Can you work these out from the model? Positions are in its coordinate system, mm. Give positions to 0.01 mm unless a question says otherwise; leave off trailing zeros. Loops run counter-clockwise (first coordinate to the right, second up) from the corner with the lowest first, then second, coordinate; pieces in that order, holes last. Notation, with made-up numbers: (33.25, -40) -> (66.25, -40) arc R23 ccw to (66.25, -16) -> close; hole circle Ø9 at (-33, 39.5). An arc over 180 degrees is marked (long way). One line per question, with ' | ' between items.
from build123d import *

# Parameters (mm, degrees)
F0_R      = 0.635
F1_DEPTH  = 3.175
F2_W      = 508
F2_H      = 25.4
F3_DEPTH  = 6.35
F4_W      = 25.4
F4_H      = 63.5
F4_H_2    = 152.4
F5_DEPTH  = 6.35
F6_W      = 508
F6_H      = 25.4
F7_DEPTH  = 6.35
F8_W      = 152.4
F8_H      = 25.4
F9_DEPTH  = 6.35
F10_W     = 25.4
F10_H     = 152.4
F11_DEPTH = 6.35
F12_W     = 25.4
F12_H     = 152.4
F13_DEPTH = 6.35
F14_W     = 76.2
F14_H     = 25.4
F15_DEPTH = 6.35


# Not quite as in the source:
# - a feature of the source that left no trace in its solid (it failed there, or was rolled back) is left out


with BuildPart() as f1:
    # F0 (on Top) → F1 (new body)
    with BuildSketch(Plane.XY):
        Polygon((285.75, -298.45), (323.85, -298.45), (577.85, -298.45), (615.95, -298.45), (1187.45, -298.45), (1276.35, -298.45), (1276.35, 298.45), (1187.45, 298.45), (285.75, 298.45), (285.75, 349.25), (361.95, 349.25), (361.95, 577.85), (285.75, 577.85), (285.75, 704.85), (-285.75, 704.85), (-285.75, 577.85), (-361.95, 577.85), (-361.95, 349.25), (-285.75, 349.25), (-285.75, 336.55), (-285.75, 298.45), (-323.85, 298.45), (-361.95, 298.45), (-577.85, 298.45), (-577.85, -298.45), (-323.85, -298.45), (-285.75, -298.45), (-285.75, -336.55), (-285.75, -622.3), (-25.4, -622.3), (-25.4, -774.7), (25.4, -774.7), (25.4, -622.3), (177.8, -622.3), (285.75, -622.3), (285.75, -336.55), align=None)
        with Locations((0, -463.55)):
            Circle(F0_R, mode=Mode.SUBTRACT)
        with Locations((-450.85, 0)):
            Circle(F0_R, mode=Mode.SUBTRACT)
        Circle(F0_R, mode=Mode.SUBTRACT)
        with Locations((0, 463.55)):
            Circle(F0_R, mode=Mode.SUBTRACT)
        with Locations((450.85, 0)):
            Circle(F0_R, mode=Mode.SUBTRACT)
        with Locations((812.8, 0)):
            Circle(F0_R, mode=Mode.SUBTRACT)
        with Locations((901.7, 0)):
            Circle(F0_R, mode=Mode.SUBTRACT)
        with Locations((990.6, 0)):
            Circle(F0_R, mode=Mode.SUBTRACT)
    extrude(amount=F1_DEPTH)

    # F2 (on face) → F3 (join)
    with BuildSketch(Plane.XY.offset(3.175)):
        with Locations((0, 679.45)):
            Rectangle(F2_W, F2_H)
    extrude(amount=F3_DEPTH)

    # F4 (on face) → F5 (join)
    with BuildSketch(Plane.XY.offset(3.175)):
        with Locations((0, -679.45)):
            Rectangle(F4_W, F4_H)
        with Locations((-323.85, 463.55)):
            Rectangle(F4_W, F4_H_2)
        with Locations((323.85, 463.55)):
            Rectangle(F4_W, F4_H_2)
    extrude(amount=F5_DEPTH)

    # F6 (on face) → F7 (join)
    with BuildSketch(Plane(origin=(0, 0, 0), x_dir=(1, 0, 0), z_dir=(0, 0, -1))):
        with Locations((901.7, -247.65)):
            Rectangle(F6_W, F6_H)
    extrude(amount=F7_DEPTH)

    # F8 (on face) → F9 (join)
    with BuildSketch(Plane(origin=(0, 0, 0), x_dir=(1, 0, 0), z_dir=(0, 0, -1))):
        with Locations((450.85, -260.35)):
            Rectangle(F8_W, F8_H)
        with Locations((-450.85, -260.35)):
            Rectangle(F8_W, F8_H)
    extrude(amount=F9_DEPTH)

    # F10 (on face) → F11 (join)
    with BuildSketch(Plane.XY.offset(3.175)):
        with Locations((1250.95, 152.4)):
            Rectangle(F10_W, F10_H)
        with Locations((1250.95, -152.4)):
            Rectangle(F10_W, F10_H)
    extrude(amount=F11_DEPTH)

    # F12 (on face) → F13 (join)
    with BuildSketch(Plane.XY):
        with Locations((-552.45, 152.4)):
            Rectangle(F12_W, F12_H)
        with Locations((-552.45, -152.4)):
            Rectangle(F12_W, F12_H)
    extrude(amount=-F13_DEPTH)

    # F14 (on face) → F15 (join)
    with BuildSketch(Plane(origin=(0, 0, 0), x_dir=(1, 0, 0), z_dir=(0, 0, -1))):
        with Locations((901.7, 247.65)):
            Rectangle(F14_W, F14_H)
    extrude(amount=F15_DEPTH)


solid = f1.part
Q1. If I drill on probe 1 along Y at (x, z) = (812.8, 1.2) (3 decimals); probe 2 along Y at (x, z) = (0, 0.7) (3 decimals); probe 3 along Z at (x, y) = (-360, -228) (3 decimals), over which ranges is the centre line in solid material (lowest first)? Write a range as from..to.
Entries:
probe 1: -298.45..-0.635, 0.635..298.45 | probe 2: -774.7..-464.185, -462.915..-0.635, 0.635..462.915, 464.185..704.85 | probe 3: 0..3.175
Q2. If we section it at C-C (x = 57.5): Write out the boundary of the cut face in (y, z) (3 decimals), plus the area to 4 significant figures.
Entries:
outline: (-622.3, 0) -> (704.85, 0) -> (704.85, 3.175) -> (692.15, 3.175) -> (692.15, 9.525) -> (666.75, 9.525) -> (666.75, 3.175) -> (-622.3, 3.175) -> close | area: 4,375 mm²
Q3. For pin 1 Ø2.5 at (x, z) = (-316, 2.5) entering from -Y; pin 2 Ø1.7 at (x, y) = (-450.85, 0) entering from +Z (3 decimals); pin 3 Ø1 at (y, z) = (641, 2) entering from -X; pin 4 Ø3 at (x, z) = (148.5, -2.5) entering from -Y, each with a flat end and sliding along its axis, tell me the tip position at first contact or that it passes through.
Entries:
pin 1: y = -298.45 | pin 2: z = 3.175 | pin 3: x = -285.75 | pin 4: through
Q4. If we section it at B-B (y = 48.5): Write out the boundary of the cut face in (x, z) (3 decimals).
Entries:
outline: (-577.85, 0) -> (1276.35, 0) -> (1276.35, 3.175) -> (-577.85, 3.175) -> close
Q5. If we section it at A-A (x = 429): Write out the boundary of the cut face in (y, z) (3 decimals), plus the area to 3 significant figures.
Entries:
outline: (-298.45, 0) -> (247.65, 0) -> (247.65, -6.35) -> (273.05, -6.35) -> (273.05, 0) -> (298.45, 0) -> (298.45, 3.175) -> (-298.45, 3.175) -> close | area: 2,060 mm²
